```python
from build123d import *

# Parameters (mm, degrees)
F0_R     = 13.208
F0_R_2   = 10.668
F1_DEPTH = 72.136
F2_R     = 13.208
F2_R_2   = 10.668
F3_DEPTH = 25.4
F4_R     = 10.255717
F5_DEPTH = 25.4
F6_R     = 10.806654
F7_DEPTH = 76.2


with BuildPart() as f1:
    # F0 (on Top) → F1 (new body)
    with BuildSketch(Plane.XY):
        Circle(F0_R)
        Circle(F0_R_2, mode=Mode.SUBTRACT)
    extrude(amount=F1_DEPTH)

    # F2 (on Right) → F3 (join)
    with BuildSketch(Plane.YZ):
        with Locations((0, 36.155518)):
            Circle(F2_R)
        with Locations((0, 36.155518)):
            Circle(F2_R_2, mode=Mode.SUBTRACT)
    extrude(amount=F3_DEPTH)

    # F4 (on Right) → F5 (cut)
    with BuildSketch(Plane.YZ):
        with Locations((0, 35.921648)):
            Circle(F4_R)
    extrude(amount=F5_DEPTH, mode=Mode.SUBTRACT)

    # F6 (on Top) → F7 (cut)
    with BuildSketch(Plane.XY):
        Circle(F6_R)
    extrude(amount=F7_DEPTH, mode=Mode.SUBTRACT)


solid = f1.part
```
Model file for the job. Use its own axes, mm. A direction names the side the tool comes from. Coordinates: 2 decimals unless noted, no trailing zeros. Order: outer loops, then holes, each group sorted by start corner. A loop starts at its lowest first (then second) coordinate and runs counter-clockwise, first axis right, second up. Notation, with made-up numbers: M 83.5,-4 L 109.5,-4 A13 ccw 109.5,4 Z; hole C 60,57 d11. An arc over 180 degrees is marked long. Answer as CSV lines item,"result".
(1) Band-saw the part on C-C, the plane z = 33. List the corners of the cut face in (x, y), then the cut area to 3 significant figures.
Geometry says:
outline,"M 3.16,-12.83 L 25.4,-12.83 L 25.4,-10.19 L 8.4,-10.19 A13.21 ccw 8.82,-9.83 L 4.49,-9.83 A10.81 cw long 4.49,9.83 L 8.82,9.83 A13.21 ccw 8.4,10.19 L 25.4,10.19 L 25.4,12.83 L 3.16,12.83 A13.21 ccw long Z"
area,"226 mm2"
(2) Wall check: line 1 along Z through (x, y) = (12.5, 0); line 2 along Y through (x, z) = (0, 44); line 3 along X through (y, z) = (7.25, 54.5). Give the ranges that are in metal, low to high.
Geometry says:
line 1,"z = 0 to 25.67, 46.18 to 72.14"
line 2,"y = -13.21 to -10.81, 10.81 to 13.21"
line 3,"x = -11.04 to -8.01, 8.01 to 11.04"
(3) Band-saw the part on B-B, the plane x = -2. List the corners of the cut face in (y, z), then the cut area to 3 significant figures.
Geometry says:
outline,"M -13.06,0 L -10.62,0 L -10.62,72.14 L -13.06,72.14 Z; M 10.62,0 L 13.06,0 L 13.06,72.14 L 10.62,72.14 Z"
area,"351 mm2"
(4) Flat gauge pins, fed straight in: pin 1 (4 mm diameter, centred on y = 3.5, z = 64.5, fed in from -X); pin 2 (1 mm diameter, centred on y = 9.5, z = 63, fed in from +X); pin 3 (6 mm diameter, centred on y = -10, z = 14, fed in from -X). Where does each tip first touch, or does it go through?
Geometry says:
pin 1,"stops at x = -13.12"
pin 2,"stops at x = 9.67"
pin 3,"stops at x = -11.2"
(5) Band-saw the part on D-D, the plane y = -9. List the corners of the cut face in (x, z).
Geometry says:
outline,"M -9.67,0 L -5.98,0 L -5.98,72.14 L -9.67,72.14 Z; M 5.98,0 L 9.67,0 L 9.67,26.49 L 25.4,26.49 L 25.4,30.43 L 9.67,30.43 L 9.67,31 L 5.98,31 Z; M 5.98,40.84 L 9.67,40.84 L 9.67,41.88 L 25.4,41.88 L 25.4,45.82 L 9.67,45.82 L 9.67,72.14 L 5.98,72.14 Z"
(6) 3-axis set-ups, long thin cutter, end or side, ignore diameter. For faces 5 (the flat face through (-11, 0, 72.136)), 6 (the cylindrical face through (15.344, -9.735, 45.082)): which of +Z, -Z, +X, -X, +Y, -Y reach the whole face in a straight line?
Geometry says:
face 5,"+Z, +X, -X, +Y, -Y"
face 6,"+X"
(7) Pull direction X, two halves, no side cores. Call faces 1 (the cylindrical face through (-13.195, 0.581, 35.563)), 2 (the cylindrical face through (18.426, 9.855, 32.07)), 3 (the flat face through (25.4, 1, 47)), 4 (the cylindrical face through (-10.796, 0.475, 35.563)): +X half, -X half, draft (parallel to the pull), parting line (faces both ways), or undercut.
Geometry says:
face 1,"parting line"
face 2,"draft"
face 3,"+X half"
face 4,"undercut"
(8) Band-saw the part on A-A, the plane y = 0. List the corners of the cut face in (x, z).
Geometry says:
outline,"M -13.21,0 L -10.81,0 L -10.81,72.14 L -13.21,72.14 Z; M 10.81,0 L 13.21,0 L 13.21,22.95 L 25.4,22.95 L 25.4,25.49 L 13.21,25.49 L 13.21,25.67 L 10.81,25.67 Z; M 10.81,46.18 L 13.21,46.18 L 13.21,46.82 L 25.4,46.82 L 25.4,49.36 L 13.21,49.36 L 13.21,72.14 L 10.81,72.14 Z"
